The listing builds one solid part. Answer for the finished solid, in the listing's coordinates (mm). A direction names the side the tool comes from. Give positions to 0.01 mm unless a question says otherwise; leave off trailing zeros. Write each loop counter-clockwise with the first axis right and the second up, starting at its lowest first coordinate (ties: lowest second). Pieces come first, ordered by that corner, then holes. Notation, with made-up numbers: (52, -12.75) -> (99, -12.75) arc R18 cw to (99, 17.25) -> close; hole circle Ø9 at (27.25, 33). An arc over 180 degrees is marked (long way). One line per question, with ' | ' between items.
from build123d import *

# Parameters (mm, degrees)
BOSS_EXTRUDE1_DEPTH = 12
SKETCH3_W           = 1.5875
SKETCH3_H           = 10
BOSS_EXTRUDE2_DEPTH = 1.5875
BOSS_EXTRUDE3_DEPTH = 1.5875


with BuildPart() as part:
    # Sketch2 → Boss-Extrude1 (new body)
    with BuildSketch(Plane.XY):
        with BuildLine():
            ThreePointArc((-7.4837, -6.930673438), (0, -10.2), (7.4837, -6.930673438))
            Line((7.4837, -6.930673438), (7.4837, -14.2875))
            Line((7.4837, -14.2875), (-7.4837, -14.2875))
            Line((-7.4837, -14.2875), (-7.4837, -6.930673438))
        make_face()
    extrude(amount=BOSS_EXTRUDE1_DEPTH)

    # Sketch3 → Boss-Extrude2 (add)
    with BuildSketch(Plane.XY.offset(12)):
        with Locations((-6.68995, -9.2875)):
            Rectangle(SKETCH3_W, SKETCH3_H)
        with Locations((6.68995, -9.2875)):
            Rectangle(SKETCH3_W, SKETCH3_H)
    extrude(amount=BOSS_EXTRUDE2_DEPTH)

    # Sketch4 → Boss-Extrude3 (add)
    with BuildSketch(Plane.XY.offset(12)):
        with BuildLine():
            Line((-5.8962, -8.323149978), (-5.8962, -14.2875))
            Line((-5.8962, -14.2875), (5.8962, -14.2875))
            Line((5.8962, -14.2875), (5.8962, -8.323149978))
            ThreePointArc((5.8962, -8.323149978), (0, -10.2), (-5.8962, -8.323149978))
        make_face()
    extrude(amount=BOSS_EXTRUDE3_DEPTH)


solid = part.part
Item 1: A tool of negligible diameter and unlimited length cuts with its end or side. For faces 1 (the face through (7, -6, 12)), 2 (the face through (0, -11, 13.588)), 3 (the face through (5.896, -6, 13)), from which of +Z, -Z, +X, -X, +Y, -Y can it reach the whole face along a straight path? Write none if from no direction.
Answers below:
face 1: -Z, +Y | face 2: +Z, +X, -X, +Y, -Y | face 3: +Z, -Z, +Y
Item 2: Find section D-D (x = -4). Write down the section's boundary in (y, z), then the cut area to 3 significant figures.
Answers below:
outline: (-14.29, 0) -> (-9.38, 0) -> (-9.38, 13.59) -> (-14.29, 13.59) -> close | area: 66.6 mm²
Item 3: Find section B-B (y = -5.75). Write down the section's boundary in (x, z), then the cut area to 3 significant figures.
Answers below:
outline: (-7.48, 12) -> (-5.9, 12) -> (-5.9, 13.59) -> (-7.48, 13.59) -> close; (5.9, 12) -> (7.48, 12) -> (7.48, 13.59) -> (5.9, 13.59) -> close | area: 5.04 mm²
Item 4: Flat-ended cylindrical pins translate along their axes: pin 1 (0.8 mm diameter, centred on x = 6.5, y = -7, fed in from -Z); pin 2 (1 mm diameter, centred on x = 1.5, z = 8.5, fed in from +Y). Find the tip coordinate at first contact, or state that the pin passes through.
Answers below:
pin 1: z = 12 | pin 2: y = -10
Item 5: Determine the mould class of faces 4 (the face through (0, -11, 0)), 5 (the face through (7.484, -10, 7)), 6 (the face through (-5.896, -6, 13)) for opening direction X: pulls with the +X half, pulls with the -X half, needs draft (parallel to the pull), parting line crosses it, or undercut.
Answers below:
face 4: needs draft | face 5: pulls with the +X half | face 6: undercut
Item 6: Find section A-A (y = -9). Write down the section's boundary in (x, z).
Answers below:
outline: (-7.48, 0) -> (-4.8, 0) -> (-4.8, 13.59) -> (-7.48, 13.59) -> close; (4.8, 0) -> (7.48, 0) -> (7.48, 13.59) -> (4.8, 13.59) -> close
Item 7: Find section C-C (z = 12.25). Write down the section's boundary in (x, y).
Answers below:
outline: (-7.48, -14.29) -> (7.48, -14.29) -> (7.48, -4.29) -> (5.9, -4.29) -> (5.9, -8.32) arc R10.2 cw to (-5.9, -8.32) -> (-5.9, -4.29) -> (-7.48, -4.29) -> close
Item 8: Consider line 1 (Z direction, x = 6, y = -8); line 2 (X direction, y = -9, z = 5.5); line 3 (X direction, y = -8, z = 10.5). Determine where each line is inside the solid, lowest interval first. Write a range as [from, to].
Answers below:
line 1: [12, 13.59] | line 2: [-7.48, -4.8], [4.8, 7.48] | line 3: [-7.48, -6.33], [6.33, 7.48]
